```python
from build123d import *

# Parameters (mm, degrees)
BOSS_EXTRUDE1_DEPTH = 1219.2
FILLET1_R           = 0.254
SKETCH4_W           = 2238.4
SKETCH4_H           = 74.945320812
CUT_EXTRUDE1_DEPTH  = 60
SKETCH8_W           = 23.813
SKETCH8_H           = 23.813
CUT_EXTRUDE6_DEPTH  = 28.313
CUT_EXTRUDE7_DEPTH  = 228.313
SKETCH10_W          = 23.813
SKETCH10_H          = 1.587
CUT_EXTRUDE8_DEPTH  = 228.313
SKETCH14_R          = 1.65
CUT_EXTRUDE11_DEPTH = 60
SKETCH15_R          = 1.65
CUT_EXTRUDE12_DEPTH = 60


with BuildPart() as part:
    # Sketch3 → Boss-Extrude1 (new, symmetric)
    with BuildSketch(Plane.XY):
        Polygon((1.5875, 25.4), (0, 25.4), (0, 0), (25.4, 0), (25.4, 1.5875), (1.5875, 1.5875), align=None)
    extrude(amount=BOSS_EXTRUDE1_DEPTH, both=True)

    # Fillet1
    fillet1_edges = [part.edges().sort_by_distance(p)[0] for p in [
        (1.5875, 1.5875, 0),
    ]]
    fillet(fillet1_edges, radius=FILLET1_R)

    # Sketch4 → Cut-Extrude1 (cut)
    with BuildSketch(Plane.ZY):
        with Locations((-100, 37.472660406)):
            Rectangle(SKETCH4_W, SKETCH4_H)
    extrude(amount=-CUT_EXTRUDE1_DEPTH, mode=Mode.SUBTRACT)

    # Sketch8 → Cut-Extrude6 (cut)
    with BuildSketch(Plane(origin=(0, 1.5875, 0), x_dir=(1, 0, 0), z_dir=(0, 1, 0))):
        with Locations((13.4935, -1207.2935)):
            Rectangle(SKETCH8_W, SKETCH8_H)
        with Locations((13.4935, -1031.1065)):
            Rectangle(SKETCH8_W, SKETCH8_H)
    extrude(amount=-CUT_EXTRUDE6_DEPTH, mode=Mode.SUBTRACT)

    # Sketch9 → Cut-Extrude7 (cut)
    with BuildSketch(Plane(origin=(0, 0, 1019.2), x_dir=(-1, 0, 0), z_dir=(0, 0, -1))):
        Polygon((-1.8415, 1.5875), (-1.587, 1.5875), (-1.5875, 1.990327362), (-1.8415, 1.990327362), align=None)
    extrude(amount=-CUT_EXTRUDE7_DEPTH, mode=Mode.SUBTRACT)

    # Sketch10 → Cut-Extrude8 (cut)
    with BuildSketch(Plane.ZY):
        with Locations((1207.2935, 0.7935)):
            Rectangle(SKETCH10_W, SKETCH10_H)
        with Locations((1031.1065, 0.7935)):
            Rectangle(SKETCH10_W, SKETCH10_H)
    extrude(amount=-CUT_EXTRUDE8_DEPTH, mode=Mode.SUBTRACT)

    # Sketch14 → Cut-Extrude11 (cut)
    with BuildSketch(Plane(origin=(0, 1.5875, 0), x_dir=(1, 0, 0), z_dir=(0, 1, 0))):
        with Locations(Location((10.3759, -1177.925, 0), (0, 0, 180))):
            Circle(SKETCH14_R)
        with Locations(Location((10.3759, -1060.4755, 0), (0, 0, 180))):
            Circle(SKETCH14_R)
        with Locations(Location((13.49375, -1079.20025, 0), (0, 0, 180))):
            Circle(SKETCH14_R)
        with Locations(Location((13.49375, -1099.20025, 0), (0, 0, 180))):
            Circle(SKETCH14_R)
        with Locations(Location((13.49375, -1119.20025, 0), (0, 0, 180))):
            Circle(SKETCH14_R)
        with Locations(Location((13.49375, -1139.20025, 0), (0, 0, 180))):
            Circle(SKETCH14_R)
        with Locations(Location((13.49375, -1159.20025, 0), (0, 0, 180))):
            Circle(SKETCH14_R)
    extrude(amount=-CUT_EXTRUDE11_DEPTH, mode=Mode.SUBTRACT)

    # Sketch15 → Cut-Extrude12 (cut)
    with BuildSketch(Plane(origin=(1.5875, 0, 0), x_dir=(0, 0, -1), z_dir=(1, 0, 0))):
        with Locations((-1184.978795667, 11.1125)):
            Circle(SKETCH15_R)
        with Locations((-1053.421204333, 11.1125)):
            Circle(SKETCH15_R)
        with Locations((-1069.2, 13.49375)):
            Circle(SKETCH15_R)
        with Locations((-1089.2, 13.49375)):
            Circle(SKETCH15_R)
        with Locations((-1109.2, 13.49375)):
            Circle(SKETCH15_R)
        with Locations((-1129.2, 13.49375)):
            Circle(SKETCH15_R)
        with Locations((-1149.2, 13.49375)):
            Circle(SKETCH15_R)
        with Locations((-1169.2, 13.49375)):
            Circle(SKETCH15_R)
    extrude(amount=-CUT_EXTRUDE12_DEPTH, mode=Mode.SUBTRACT)


solid = part.part
```
CAD build for the part. Positions are in the model's coordinates, mm. A direction names the side the tool comes from. Round coordinates to 2 decimals unless told otherwise and drop trailing zeros. Write each loop counter-clockwise with the first axis right and the second up, starting at its lowest first coordinate (ties: lowest second). Pieces come first, ordered by that corner, then holes.
Item 1: Band-saw the part on A-A on z = 1089.2. Write the cut outline in (x, y).
Filled in:
outline: (0, 0) - (25.4, 0) - (25.4, 1.59) - (1.59, 1.59) - (1.59, 1.99) - (1.59, 11.84) - (0, 11.84) - close; (0, 15.14) - (1.59, 15.14) - (1.59, 25.4) - (0, 25.4) - close
Item 2: Drill centre lines: L1, parallel to Y at x = 1.15, z = 1109.2; L2, parallel to X at y = 22, z = 1153.5. Where is each one in solid material? Low to high.
Filled in:
L1: y = 0 to 11.84, 15.14 to 25.4
L2: x = 0 to 1.59
Item 3: Band-saw the part on D-D on x = 18.75. Write the cut outline in (y, z), then the cut area to 3 significant figures.
Filled in:
outline: (0, 1043.01) - (1.59, 1043.01) - (1.59, 1195.39) - (0, 1195.39) - close
area: 242 mm2
Item 4: Tool access for faces 1 (the cylindrical face through (0.8, 13.57, 1090.85)), 2 (the flat face through (11, 1.588, 1118)): list every direction of +Z, -Z, +X, -X, +Y, -Y with a clear straight run to the whole face (end or side of a thin tool).
Filled in:
face 1: +X, -X
face 2: +Z, -Z, +X, +Y
Item 5: Band-saw the part on C-C on z = 1115.5. Write the cut outline in (x, y).
Filled in:
outline: (0, 0) - (25.4, 0) - (25.4, 1.59) - (1.59, 1.59) - (1.59, 1.99) - (1.59, 25.4) - (0, 25.4) - close
Item 6: Band-saw the part on B-B on y = 17.5. Write the cut outline in (x, z), then the cut area to 4 significant figures.
Filled in:
outline: (0, 1019.2) - (1.59, 1019.2) - (1.59, 1219.2) - (0, 1219.2) - close
area: 317.5 mm2
Item 7: Drop flat-ended pins along their axis: pin 1 Ø8 at (y, z) = (14, 1189.5) entering from +X; pin 2 Ø0.8 at (x, z) = (0.5, 1202.5) entering from -Y; pin 3 Ø5.5 at (x, z) = (13.49, 1119.2) entering from +Y. Give the stop position or say it passes through.
Filled in:
pin 1: stops at x = 1.59
pin 2: stops at y = 1.59
pin 3: stops at y = 1.59
Item 8: Mould opens along X. For faces 3 (the cylindrical face through (10.59, 0.8, 1062.11)), 4 (the cylindrical face through (0.8, 13.57, 1150.85)), 5 (the flat face through (0, 13, 1121)) say: released by +X, released by -X, zero draft, split by the parting line, or undercut.
Filled in:
face 3: undercut
face 4: zero draft
face 5: released by -X
